from build123d import *

# Parameters (mm, degrees)
F1_DEPTH = 3.175


with BuildPart() as f1:
    # F0 (on Front) → F1 (new body)
    with BuildSketch(Plane.XZ):
        Polygon((-241.3, 368.3), (-241.3, 342.9), (-215.9, 342.9), (215.9, 342.9), (241.3, 342.9), (241.3, 368.3), align=None)
        Polygon((-215.9, 342.9), (-241.3, 342.9), (-241.3, -342.9), (-215.9, -342.9), (-215.9, -317.5), align=None)
        Polygon((215.9, -317.5), (-215.9, -317.5), (-215.9, -342.9), (0, -342.9), (215.9, -342.9), align=None)
        Polygon((241.3, 342.9), (215.9, 342.9), (215.9, -317.5), (215.9, -342.9), (241.3, -342.9), align=None)
    extrude(amount=F1_DEPTH)


solid = f1.part
Source: CAD feature listing. Evaluate the final solid. Frame: model axes, mm. Coordinates: 2 decimals unless noted, no trailing zeros. Write each loop counter-clockwise with the first axis right and the second up, starting at its lowest first coordinate (ties: lowest second). Pieces come first, ordered by that corner, then holes. Notation, with made-up numbers: M 6,41.5 L 12,41.5 A14 cw 12,58.5 Z; hole C -13.5,21.5 d11. An arc over 180 degrees is marked long. Use a Markdown table: item, result.
1) Section B-B, the plane z = 19. Output: boundary loops of the cut face in (x, y) (3 decimals), then the cut area to 3 significant figures.
Conclusion:
| item | result |
|---|---|
| outline | M -241.3,-3.175 L -215.9,-3.175 L -215.9,0 L -241.3,0 Z; M 215.9,-3.175 L 241.3,-3.175 L 241.3,0 L 215.9,0 Z |
| area | 161 mm^2 |
2) Section C-C, the plane y = -0.8. Output: boundary loops of the cut face in (x, z), then the cut area to 3 significant figures.
Conclusion:
| item | result |
|---|---|
| outline | M -241.3,-342.9 L 241.3,-342.9 L 241.3,368.3 L -241.3,368.3 Z; hole M -215.9,-317.5 L 215.9,-317.5 L 215.9,342.9 L -215.9,342.9 Z |
| area | 58,100 mm^2 |
3) Section A-A, the plane x = 143. Output: boundary loops of the cut face in (y, z) (3 decimals).
Conclusion:
| item | result |
|---|---|
| outline | M -3.175,-342.9 L 0,-342.9 L 0,-317.5 L -3.175,-317.5 Z; M -3.175,342.9 L 0,342.9 L 0,368.3 L -3.175,368.3 Z |
4) Ray query, L1, parallel to Z at x = -154, y = -2; L2, parallel to X at y = -2.85, z = -195. Return the intervals inside material, ascending.
Conclusion:
| item | result |
|---|---|
| L1 | z = -342.9 to -317.5, 342.9 to 368.3 |
| L2 | x = -241.3 to -215.9, 215.9 to 241.3 |
